Geometry: final body of the model. Coordinates: model frame, mm. Give positions to 0.01 mm unless a question says otherwise; leave off trailing zeros. Loops run counter-clockwise (first coordinate to the right, second up) from the corner with the lowest first, then second, coordinate; pieces in that order, holes last. Notation, with made-up numbers: (48, -5.75) -> (105, -5.75) arc R32 cw to (105, 20.25) -> close; hole circle Ø4 at (12.5, 22). An arc over 180 degrees is marked (long way). Answer in a Markdown table with one row per item. Add a question column.
1) First-contact query: P1, Ø6, axis at x = 49, y = -29.5, coming from the +Z side; P2, Ø9.5, axis at x = 30, y = 25, coming from the +Z side; P3, Ø6, axis at y = 1.5, z = 14, coming from the -X side (3 decimals); P4, Ø3.5, axis at x = -85, y = -25, coming from the +Z side. Flat tips, straight axial feed; report the tip coordinate or a pass-through.
2) Line query: line 1 (X direction, y = -13, z = 2.25); line 2 (Y direction, x = -30, z = 3.9); line 3 (Y direction, x = -71.5, z = 9.5). Output: solid intervals per line, ascending. Write a range as from..to.
3) Section query B-B (y = -2). Return the cut outline in (x, z).
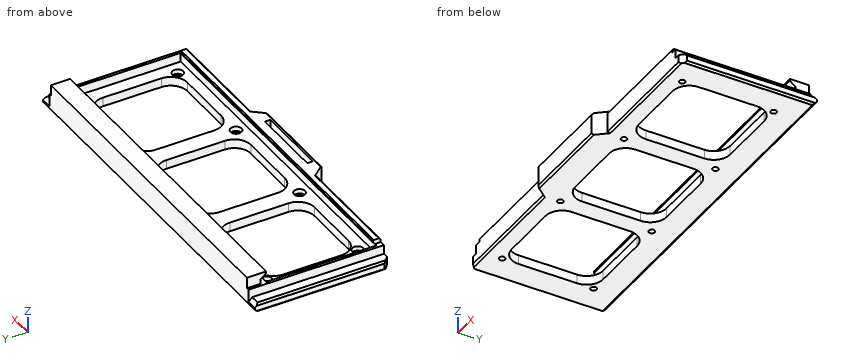
```python
from build123d import *

# Parameters (mm, degrees)
SKETCH_W        = 200
SKETCH_H        = 80
PAD_DEPTH       = 5
SKETCH001_W     = 200
SKETCH001_H     = 80
SKETCH001_W_2   = 185
SKETCH001_H_2   = 60.5
PAD001_DEPTH    = 5
SKETCH002_W     = 185
SKETCH002_H     = 10.5
PAD002_DEPTH    = 6
SKETCH003_W     = 182
SKETCH003_H     = 10.25
PAD003_DEPTH    = 2.5
POCKET_DEPTH    = 192.501
SKETCH005_R     = 1.6
POCKET001_DEPTH = 5
SKETCH006_R     = 3
POCKET002_DEPTH = 2.5
SKETCH007_W     = 6
SKETCH007_H     = 80
POCKET003_DEPTH = 5
CHAMFER_SIZE    = 2
SKETCH008_W     = 40
SKETCH008_H     = 3
POCKET004_DEPTH = 5
POCKET005_DEPTH = 12.501
CHAMFER001_SIZE = 3
CHAMFER002_SIZE = 1
CHAMFER003_SIZE = 1
CHAMFER004_SIZE = 1
CHAMFER005_SIZE = 1.24
CHAMFER006_SIZE = 0.5


with BuildPart() as part:
    # Sketch → Pad (new body)
    with BuildSketch(Plane.XY):
        Rectangle(SKETCH_W, SKETCH_H)
    extrude(amount=PAD_DEPTH)

    # Sketch001 (on Face6 of Pad) → Pad001 (join)
    with BuildSketch(Plane.XY.offset(5)):
        Rectangle(SKETCH001_W, SKETCH001_H)
        with Locations((0, -0.75)):
            Rectangle(SKETCH001_W_2, SKETCH001_H_2, mode=Mode.SUBTRACT)
    extrude(amount=PAD001_DEPTH)

    # Sketch002 (on Face3 of Pad001) → Pad002 (join)
    with BuildSketch(Plane.XY.offset(10)):
        with Locations((0, 34.75)):
            Rectangle(SKETCH002_W, SKETCH002_H)
    extrude(amount=PAD002_DEPTH)

    # Sketch003 (on Face5 of Pad002) → Pad003 (join)
    with BuildSketch(Plane.XY.offset(10)):
        with Locations((0, -34.875)):
            Rectangle(SKETCH003_W, SKETCH003_H)
    extrude(amount=PAD003_DEPTH)

    # Sketch004 (on Face7 of Pad003) → Pocket (cut, through all)
    with BuildSketch(Plane(origin=(-92.5, 0, 0), x_dir=(0, -1, 0), z_dir=(-1, 0, 0))):
        Polygon((-32.5, 12.5), (-32.5, 10), (-29.5, 10), (-29.5, 15), align=None)
    extrude(amount=-POCKET_DEPTH, mode=Mode.SUBTRACT)

    # Sketch005 (on Face21 of Pocket) → Pocket001 (cut)
    with BuildSketch(Plane.XY.offset(5)):
        with Locations((-85, -25)):
            Circle(SKETCH005_R)
        with Locations((-30, -25)):
            Circle(SKETCH005_R)
        with Locations((30, -25)):
            Circle(SKETCH005_R)
        with Locations((85, -25)):
            Circle(SKETCH005_R)
        with Locations((85, 25)):
            Circle(SKETCH005_R)
        with Locations((30, 25)):
            Circle(SKETCH005_R)
        with Locations((-30, 25)):
            Circle(SKETCH005_R)
        with Locations((-85, 25)):
            Circle(SKETCH005_R)
        with BuildLine():
            Line((-25, 16), (-25, -16))
            ThreePointArc((-25, -16), (-22.363961, -22.363961), (-16, -25))
            Line((-16, -25), (16, -25))
            ThreePointArc((16, -25), (22.363961, -22.363961), (25, -16))
            Line((25, -16), (25, 16))
            ThreePointArc((25, 16), (22.363961, 22.363961), (16, 25))
            Line((16, 25), (-16, 25))
            ThreePointArc((-16, 25), (-22.363961, 22.363961), (-25, 16))
        make_face()
        with BuildLine():
            Line((-85, 16), (-85, -16))
            ThreePointArc((-85, -16), (-82.363961, -22.363961), (-76, -25))
            Line((-76, -25), (-44, -25))
            ThreePointArc((-44, -25), (-37.636039, -22.363961), (-35, -16))
            Line((-35, -16), (-35, 16))
            ThreePointArc((-35, 16), (-37.636039, 22.363961), (-44, 25))
            Line((-44, 25), (-76, 25))
            ThreePointArc((-76, 25), (-82.363961, 22.363961), (-85, 16))
        make_face()
        with BuildLine():
            Line((35, 16), (35, -16))
            ThreePointArc((35, -16), (37.636039, -22.363961), (44, -25))
            Line((44, -25), (76, -25))
            ThreePointArc((76, -25), (82.363961, -22.363961), (85, -16))
            Line((85, -16), (85, 16))
            ThreePointArc((85, 16), (82.363961, 22.363961), (76, 25))
            Line((76, 25), (44, 25))
            ThreePointArc((44, 25), (37.636039, 22.363961), (35, 16))
        make_face()
    extrude(amount=-POCKET001_DEPTH, mode=Mode.SUBTRACT)

    # Sketch006 (on Face45 of Pocket001) → Pocket002 (cut)
    with BuildSketch(Plane.XY.offset(5)):
        with Locations((-85, 25)):
            Circle(SKETCH006_R)
        with Locations((-85, -25)):
            Circle(SKETCH006_R)
        with Locations((-30, -25)):
            Circle(SKETCH006_R)
        with Locations((-30, 25)):
            Circle(SKETCH006_R)
        with Locations((30, 25)):
            Circle(SKETCH006_R)
        with Locations((30, -25)):
            Circle(SKETCH006_R)
        with Locations((85, -25)):
            Circle(SKETCH006_R)
        with Locations((85, 25)):
            Circle(SKETCH006_R)
    extrude(amount=-POCKET002_DEPTH, mode=Mode.SUBTRACT)

    # Sketch007 (on Face38 of Pocket002) → Pocket003 (cut)
    with BuildSketch(Plane.XY.offset(10)):
        with Locations((-97, 0)):
            Rectangle(SKETCH007_W, SKETCH007_H)
        with Locations((97, 0)):
            Rectangle(SKETCH007_W, SKETCH007_H)
    extrude(amount=-POCKET003_DEPTH, mode=Mode.SUBTRACT)

    # Chamfer
    chamfer_edges = [part.edges().sort_by_distance(p)[0] for p in [
        (-97, 40, 5),
        (0, 40, 0),
        (97, 40, 5),
    ]]
    chamfer(chamfer_edges, length=CHAMFER_SIZE)

    # Sketch008 (on Face44 of Chamfer) → Pocket004 (cut)
    with BuildSketch(Plane.XY.offset(12.5)):
        with Locations((0, -36.5)):
            Rectangle(SKETCH008_W, SKETCH008_H)
    extrude(amount=-POCKET004_DEPTH, mode=Mode.SUBTRACT)

    # Sketch009 (on Face44 of Pocket004) → Pocket005 (cut, through all)
    with BuildSketch(Plane.XY.offset(12.5)):
        Polygon((-100, -34), (-100, -40), (-25, -40), (-30, -34), align=None)
        Polygon((30, -34), (25, -40), (100, -40), (100, -34), align=None)
    extrude(amount=-POCKET005_DEPTH, mode=Mode.SUBTRACT)

    # Chamfer001
    chamfer001_edges = [part.edges().sort_by_distance(p)[0] for p in [
        (-100, -34, 2.5),
        (100, -34, 2.5),
    ]]
    chamfer(chamfer001_edges, length=CHAMFER001_SIZE)

    # Chamfer002
    chamfer002_edges = [part.edges().sort_by_distance(p)[0] for p in [
        (-60.5, -34, 12.5),
        (-63.5, -34, 0),
        (60.5, -34, 12.5),
        (63.5, -34, 0),
    ]]
    chamfer(chamfer002_edges, length=CHAMFER002_SIZE)

    # Chamfer003
    chamfer003_edges = [part.edges().sort_by_distance(p)[0] for p in [
        (0, -40, 12.5),
        (0, -40, 0),
    ]]
    chamfer(chamfer003_edges, length=CHAMFER003_SIZE)

    # Chamfer004
    chamfer004_edges = [part.edges().sort_by_distance(p)[0] for p in [
        (100, 3.5, 5),
        (100, 3.5, 0),
        (-100, 3.5, 5),
        (-100, 3.5, 0),
    ]]
    chamfer(chamfer004_edges, length=CHAMFER004_SIZE)

    # Chamfer005
    chamfer005_edges = [part.edges().sort_by_distance(p)[0] for p in [
        (0, -29.75, 10),
    ]]
    chamfer(chamfer005_edges, length=CHAMFER005_SIZE)

    # Chamfer006
    chamfer006_edges = [part.edges().sort_by_distance(p)[0] for p in [
        (0, -29.75, 12.5),
    ]]
    chamfer(chamfer006_edges, length=CHAMFER006_SIZE)


solid = part.part
```
Evaluation:
| question | item | result |
|---|---|---|
| 1 | P1 | z = 12.5 |
| 1 | P2 | z = 16 |
| 1 | P3 | through |
| 1 | P4 | z = 2.5 |
| 2 | line 1 | -100..-85, -35..-25, 25..35, 85..100 |
| 2 | line 2 | -34..-28, -22..22, 28..40 |
| 2 | line 3 | -34..-31, 29.5..40 |
| 3 | outline | (-100, 1) -> (-99, 0) -> (-85, 0) -> (-85, 5) -> (-92.5, 5) -> (-92.5, 10) -> (-94, 10) -> (-94, 5) -> (-99, 5) -> (-100, 4) -> close; (-35, 0) -> (-25, 0) -> (-25, 5) -> (-35, 5) -> close; (25, 0) -> (35, 0) -> (35, 5) -> (25, 5) -> close; (85, 0) -> (99, 0) -> (100, 1) -> (100, 4) -> (99, 5) -> (94, 5) -> (94, 10) -> (92.5, 10) -> (92.5, 5) -> (85, 5) -> close |
